from build123d import *

# Parameters (mm, degrees)
CUT_EXTRUDE1_START = 1.4986
CUT_EXTRUDE1_DEPTH = 10.922
CIRPATTERN1_COUNT  = 20
SKETCH4_R          = 1.5875
CUT_EXTRUDE2_DEPTH = 30.142626104
CUT_EXTRUDE3_DEPTH = 1.190625
CIRPATTERN2_COUNT  = 2
CIRPATTERN2_ANGLE  = 90


with BuildPart() as part:
    # Sketch2 → Revolve1 (revolve)
    with BuildSketch(Plane(origin=(0, 0, 0), x_dir=(0, 0, -1), z_dir=(1, 0, 0)), mode=Mode.PRIVATE) as revolve1_sk:
        with BuildLine():
            Line((-11.1125, 3.175), (11.1125, 3.175))
            Line((11.1125, 3.175), (11.1125, 19.05))
            Line((11.1125, 19.05), (10.26795, 19.05))
            ThreePointArc((10.26795, 19.05), (9.646555263, 18.316132165), (9.4234, 17.380773865))
            Line((9.4234, 17.380773865), (9.4234, 15.711547731))
            Line((9.4234, 15.711547731), (-1.4986, 15.711547731))
            Line((-1.4986, 15.711547731), (-1.4986, 17.380773865))
            ThreePointArc((-1.4986, 17.380773865), (-1.721755263, 18.316132165), (-2.34315, 19.05))
            Line((-2.34315, 19.05), (-3.1877, 19.05))
            Line((-3.1877, 19.05), (-3.1877, 11.8999))
            Line((-3.1877, 11.8999), (-11.1125, 11.8999))
            Line((-11.1125, 11.8999), (-11.1125, 3.175))
        make_face()
    revolve(revolve1_sk.sketch.rotate(Axis((0, 0, 11.1125), (0, 0, -1)), 90), axis=Axis((0, 0, 11.1125), (0, 0, -1)))

    # Sketch3 → Cut-Extrude1 (cut)
    with BuildSketch(Plane.XY.offset(CUT_EXTRUDE1_START)):
        with BuildLine():
            Line((-0.690489274, 14.3891), (0.690489274, 14.3891))
            Line((0.690489274, 14.3891), (1.2827, 15.6591))
            ThreePointArc((1.2827, 15.6591), (0, 15.711547731), (-1.2827, 15.6591))
            Line((-1.2827, 15.6591), (-0.690489274, 14.3891))
        make_face()
    cut_extrude1 = extrude(amount=-CUT_EXTRUDE1_DEPTH, mode=Mode.SUBTRACT)

    # CirPattern1: Cut-Extrude1 ×20 about axis
    cirpattern1_axis = Axis((0, 0, 0), (0, 0, 1))
    for i in range(1, CIRPATTERN1_COUNT):
        add(cut_extrude1.rotate(cirpattern1_axis, i * 360 / CIRPATTERN1_COUNT), mode=Mode.SUBTRACT)

    # Sketch4 → Cut-Extrude2 (cut, through all)
    with BuildSketch(Plane(origin=(0, 0, 0), x_dir=(1, 0, 0), z_dir=(0, 1, 0))):
        with Locations(Location((0, -7.1501, 0), (0, 0, 90))):
            Circle(SKETCH4_R)
    cut_extrude2 = extrude(amount=CUT_EXTRUDE2_DEPTH, mode=Mode.SUBTRACT)

    # Sketch5 → Revolve2 (revolve)
    with BuildSketch(Plane.XY.offset(7.1501), mode=Mode.PRIVATE) as revolve2_sk:
        Polygon((0, 11.793534829), (0, 3.175), (-0.9525, 3.175), (-1.5875, 3.81), (-1.5875, 11.158534829), (-0.9525, 11.793534829), align=None)
    revolve2 = revolve(revolve2_sk.sketch.rotate(Axis((0, 0, 7.1501), (0, 1, 0)), 270), axis=Axis((0, 0, 7.1501), (0, 1, 0)))

    # Sketch6 → Cut-Extrude3 (cut)
    with BuildSketch(Plane(origin=(0, 11.793534829, 0), x_dir=(-1, 0, 0), z_dir=(0, -1, 0))):
        Polygon((0, -6.233556448), (-0.79375, -6.691828224), (-0.79375, -7.608371776), (0, -8.066643552), (0.79375, -7.608371776), (0.79375, -6.691828224), align=None)
    cut_extrude3 = extrude(amount=CUT_EXTRUDE3_DEPTH, mode=Mode.SUBTRACT)

    # CirPattern2: Cut-Extrude2, Revolve2, Cut-Extrude3 ×2 about axis
    cirpattern2_axis = Axis((0, 0, 0), (0, 0, -1))
    add([cut_extrude2.rotate(cirpattern2_axis, i * CIRPATTERN2_ANGLE / (CIRPATTERN2_COUNT - 1)) for i in range(1, CIRPATTERN2_COUNT)], mode=Mode.SUBTRACT)
    add([revolve2.rotate(cirpattern2_axis, i * CIRPATTERN2_ANGLE / (CIRPATTERN2_COUNT - 1)) for i in range(1, CIRPATTERN2_COUNT)])
    add([cut_extrude3.rotate(cirpattern2_axis, i * CIRPATTERN2_ANGLE / (CIRPATTERN2_COUNT - 1)) for i in range(1, CIRPATTERN2_COUNT)], mode=Mode.SUBTRACT)


solid = part.part
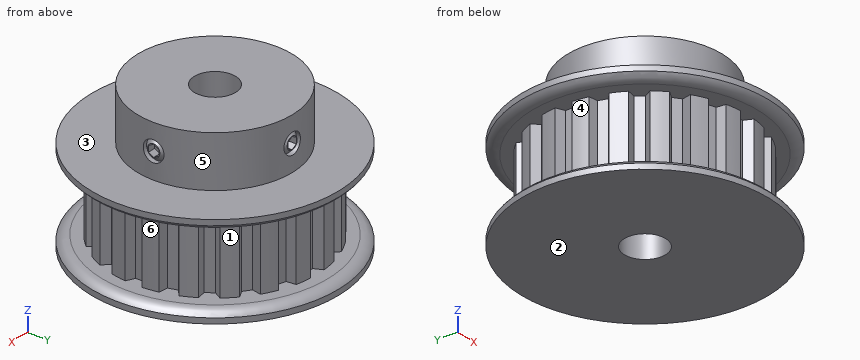
Build history of the part. All positions in model axes, mm. Face numbers are marked on the shaded views. A direction names the side the tool comes from. Coordinates: 2 decimals unless noted, no trailing zeros. One line per item, written item: value.
(1) Probe line 1 (Z direction, x = 0, y = 11); line 2 (X direction, y = 3.5, z = 7.25); line 3 (X direction, y = -14, z = -2). List the from-to ranges inside material, lowest first. Write a range as [from, to].
Checked values:
line 1: [-11.11, 6.23], [8.07, 11.11]
line 2: [-11.37, -1.58], [-1.27, 1.27], [1.58, 11.37]
line 3: [-7.13, -5.6], [-3.78, 3.78], [5.6, 7.13]
(2) Drop flat-ended pins along their axis: pin 1 Ø1 at (y, z) = (11.5, 7) entering from -X; pin 2 Ø1.1 at (x, z) = (0, -3.5) entering from -Y; pin 3 Ø1.5 at (y, z) = (-11.5, -4.5) entering from -X. Give the stop position or say it passes through.
Checked values:
pin 1: x = -4.54
pin 2: y = -14.39
pin 3: x = -11.46
(3) Mould opens along Z. For the marked faces 1, 2 and 3 say: pulls with the +Z half, pulls with the -Z half, needs draft (parallel to the pull), parting line crosses it, or undercut.
Checked values:
face 1: undercut
face 2: pulls with the -Z half
face 3: pulls with the +Z half
(4) Tool access for the marked faces 4, 5 and 6: list every direction of +Z, -Z, +X, -X, +Y, -Y with a clear straight run to the whole face (end or side of a thin tool).
Checked values:
face 4: -X, -Y
face 5: +Z
face 6: +X, +Y
